Geometry: final body of the model. Coordinates: model frame, mm. Face numbers are marked on the shaded views. A direction names the side the tool comes from. Give positions to 0.01 mm unless a question says otherwise; leave off trailing zeros. Order: outer loops, then holes, each group sorted by start corner. A loop starts at its lowest first (then second) coordinate and runs counter-clockwise, first axis right, second up. Notation, with made-up numbers: (11.25, 17) -> (20.25, 17) arc R19 ccw to (20.25, 23) -> close; hole circle Ø4 at (-36.5, 67). An arc over 180 degrees is marked (long way). Write item = value, one per line.
```python
from build123d import *

# Parameters (mm, degrees)
EXTRUDE_1_DEPTH = 10
SKETCH_2_W      = 14
SKETCH_2_H      = 10
SKETCH_2_R      = 2.6
EXTRUDE_2_DEPTH = 4
FILLET_1_R      = 3


with BuildPart() as part:
    # 草图1 → 凸台-拉伸1 (new body)
    with BuildSketch(Plane(origin=(0, 0, 0), x_dir=(1, 0, 0), z_dir=(0, 1, 0))):
        with BuildLine():
            Line((-23, 0), (-23, -36.75))
            Line((-23, -36.75), (-20, -36.75))
            Line((-20, -36.75), (-20, 0))
            ThreePointArc((-20, 0), (0, 20), (20, 0))
            Line((20, 0), (20, -36.75))
            Line((20, -36.75), (23, -36.75))
            Line((23, -36.75), (23, 0))
            ThreePointArc((23, 0), (0, 23), (-23, 0))
        make_face()
    extrude(amount=EXTRUDE_1_DEPTH)

    # 草图2 → 凸台-拉伸2 (add)
    # profile 1 of 2: a face of its own
    with BuildSketch(Plane.XY.offset(36.75)):
        with Locations((-30, 5)):
            Rectangle(SKETCH_2_W, SKETCH_2_H)
        with Locations((-30, 5)):
            Circle(SKETCH_2_R, mode=Mode.SUBTRACT)
    # profile 2 of 2: a face of its own
    with BuildSketch(Plane.XY.offset(36.75)):
        with Locations((30, 5)):
            Rectangle(SKETCH_2_W, SKETCH_2_H)
        with Locations(Location((30, 5, 0), (0, 0, 180))):
            Circle(SKETCH_2_R, mode=Mode.SUBTRACT)
    extrude(amount=-EXTRUDE_2_DEPTH)

    # 圆角1
    fillet_1_edges = [part.edges().sort_by_distance(p)[0] for p in [
        (-23, 5, 32.75),
        (23, 5, 32.75),
    ]]
    fillet(fillet_1_edges, radius=FILLET_1_R)


solid = part.part
```
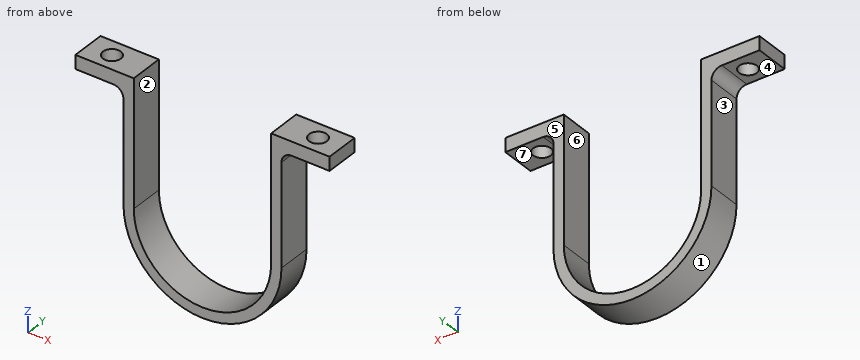
1) Section query A-A (y = 5). Output: boundary loops of the cut face in (x, z).
Check sheet entries:
outline = (-37, 32.75) -> (-32.6, 32.75) -> (-32.6, 36.75) -> (-37, 36.75) -> close; (-27.4, 32.75) -> (-26, 32.75) arc R3 cw to (-23, 29.75) -> (-23, 0) arc R23 ccw to (23, 0) -> (23, 29.75) arc R3 cw to (26, 32.75) -> (27.4, 32.75) -> (27.4, 36.75) -> (20, 36.75) -> (20, 0) arc R20 cw to (-20, 0) -> (-20, 36.75) -> (-27.4, 36.75) -> close; (32.6, 32.75) -> (37, 32.75) -> (37, 36.75) -> (32.6, 36.75) -> close
2) Section query C-C (z = 11). Output: boundary loops of the cut face in (x, y), plus the area to 3 significant figures.
Check sheet entries:
outline = (-23, 0) -> (-20, 0) -> (-20, 10) -> (-23, 10) -> close; (20, 0) -> (23, 0) -> (23, 10) -> (20, 10) -> close
area = 60.0 mm²
3) Line query: line 1 (X direction, y = 2.5, z = 20.5); line 2 (Y direction, x = -30, z = 34.95); line 3 (Z direction, x = 26, y = 8.5). Output: solid intervals per line, ascending. Write a range as from..to.
Check sheet entries:
line_1 = -23..-20, 20..23
line_2 = 0..2.4, 7.6..10
line_3 = 32.75..36.75
4) Section query D-D (x = 0). Output: boundary loops of the cut face in (y, z).
Check sheet entries:
outline = (0, -23) -> (10, -23) -> (10, -20) -> (0, -20) -> close
5) Reachability of the marked faces 5, 6 and 7 from +Z, -Z, +X, -X, +Y, -Y: full face, straight path, thin tool, end or side. Return the list, or none.
Check sheet entries:
face_5 = +Z, -Z, +X, -X, +Y
face_6 = +Z, +Y, -Y
face_7 = -Z, +X, +Y, -Y
6) Mould query, pull axis X, two halves, no side actions, for the marked faces 1, 2, 3 and 4. Classes: +X half, -X half, draft (parallel to the pull), parting line (faces both ways), or undercut.
Check sheet entries:
face_1 = parting line
face_2 = undercut
face_3 = -X half
face_4 = draft
7) Section query B-B (x = 30). Output: boundary loops of the cut face in (y, z).
Check sheet entries:
outline = (0, 32.75) -> (2.4, 32.75) -> (2.4, 36.75) -> (0, 36.75) -> close; (7.6, 32.75) -> (10, 32.75) -> (10, 36.75) -> (7.6, 36.75) -> close
8) First-contact query: P1, Ø6, axis at x = -11, y = 1.5, coming from the -Z side; P2, Ø3, axis at x = -5, y = 5.5, coming from the +Z side; P3, Ø5, axis at y = 3, z = 16, coming from the -X side; P4, Ø3, axis at x = 30, y = 5, coming from the -Z side. Flat tips, straight axial feed; report the tip coordinate or a pass-through.
Check sheet entries:
P1 = -21.56
P2 = -18.91
P3 = -23
P4 = through
